Can you work these out from the drawing? Everything is in mm from the part's minimum corner. Round coordinates to 2 decimals unless told otherwise and drop trailing zeros. Write each loop counter-clockwise with the first axis right and the second up, starting at its lowest first coordinate (ties: lowest second). Pieces come first, ordered by that corner, then holes. Notation, with made-up numbers: (10.5, 25) -> (15.5, 25) arc R11 ccw to (15.5, 31) -> close; hole circle Ø6 at (60, -7). An arc over 180 degrees is marked (long way). Put each result on its own line as item: value. Start each with the question number.
1. Suppose I cut it at B-B (z = 5.75). Please give me the cut outline in (x, y) (3 decimals).
2. Suppose I cut it at C-C (y = 4). Please give me the cut outline in (x, z).
3. I need wall thicknesses on probe 1 along Y at (x, z) = (12, 11.25); probe 2 along Y at (x, z) = (38.5, 22.25); probe 3 along Y at (x, z) = (6, 11.5). Which ranges of each line are inside material? Lowest first, please. Write a range as from..to.
4. Suppose I cut it at A-A (x = 38). Please give me the cut outline in (y, z).
5. Suppose I cut it at D-D (x = 5). Please give me the cut outline in (y, z).
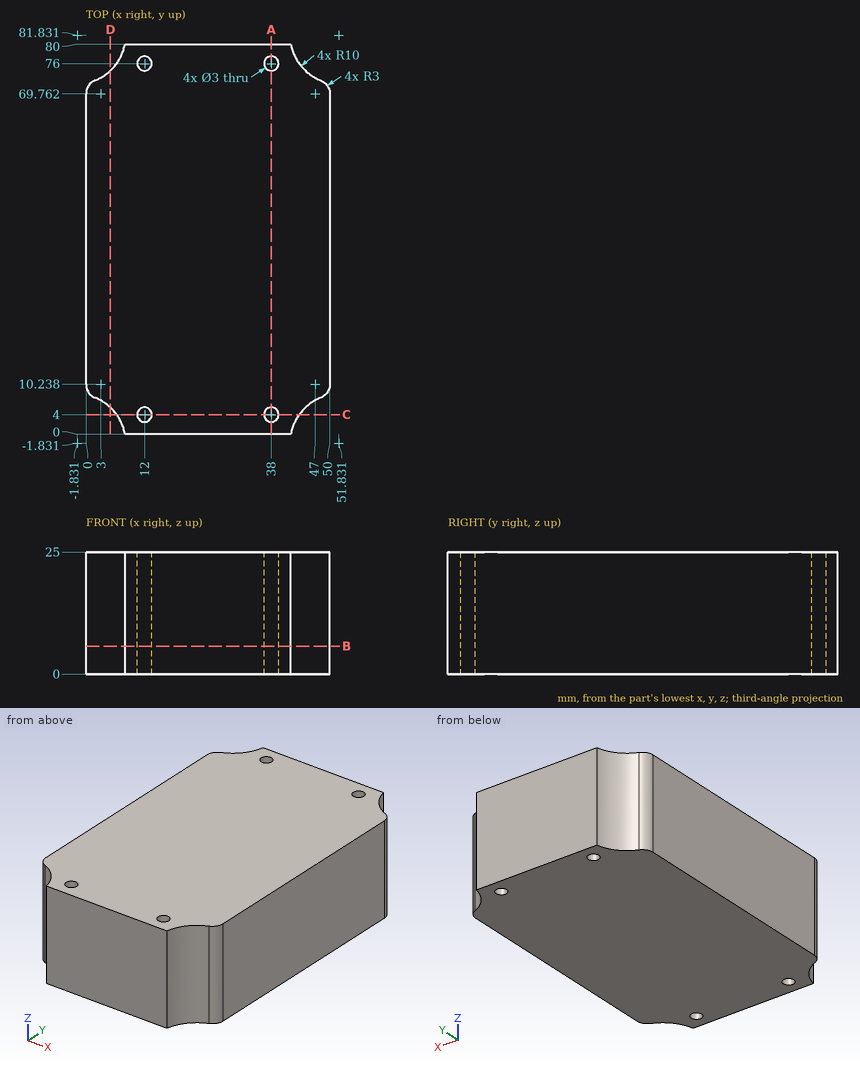
Verdict:
1. outline: (0, 10.238) arc R3 ccw to (1.885, 7.453) arc R10 cw to (8, 0) -> (42, 0) arc R10 cw to (48.115, 7.453) arc R3 ccw to (50, 10.238) -> (50, 69.762) arc R3 ccw to (48.115, 72.547) arc R10 cw to (42, 80) -> (8, 80) arc R10 cw to (1.885, 72.547) arc R3 ccw to (0, 69.762) -> close; hole circle Ø3 at (12, 4); hole circle Ø3 at (12, 76); hole circle Ø3 at (38, 4); hole circle Ø3 at (38, 76)
2. outline: (6.29, 0) -> (10.5, 0) -> (10.5, 25) -> (6.29, 25) -> close; (13.5, 0) -> (36.5, 0) -> (36.5, 25) -> (13.5, 25) -> close; (39.5, 0) -> (43.71, 0) -> (43.71, 25) -> (39.5, 25) -> close
3. probe 1: y = 0..2.5, 5.5..74.5, 77.5..80
3. probe 2: y = 0..2.59, 5.41..74.59, 77.41..80
3. probe 3: y = 4.39..75.61
4. outline: (0, 0) -> (2.5, 0) -> (2.5, 25) -> (0, 25) -> close; (5.5, 0) -> (74.5, 0) -> (74.5, 25) -> (5.5, 25) -> close; (77.5, 0) -> (80, 0) -> (80, 25) -> (77.5, 25) -> close
5. outline: (5.47, 0) -> (74.53, 0) -> (74.53, 25) -> (5.47, 25) -> close
